Geometry: final body of the model. Coordinates: model frame, mm. A direction names the side the tool comes from. Coordinates: 2 decimals unless noted, no trailing zeros. Write each loop counter-clockwise with the first axis right and the second up, starting at its lowest first coordinate (ties: lowest second). Pieces come first, ordered by that corner, then holes. Notation, with made-up numbers: M 64,31 L 86,31 A10 ccw 86,35 Z; hole C 80.5,-11 d5. An arc over 180 degrees is marked long. Write item = value, one per line. Start each with the question number.
Item 1: Section C-C on x = 58. Output: boundary loops of the cut face in (y, z), plus the area to 3 significant figures.
Item 2: First-contact query: pin 1 Ø0.7 at (x, z) = (71, 1) entering from -Y; pin 2 Ø0.7 at (x, z) = (59.5, 1) entering from +Y; pin 3 Ø1.7 at (y, z) = (-13, -1) entering from +X. Flat tips, straight axial feed; report the tip coordinate or a pass-through.
Item 3: Section B-B on x = 8. Output: boundary loops of the cut face in (y, z), plus the area to 3 significant figures.
Item 4: Pull-direction query (X, two-part tool) for faces 1 (the flat face through (65, -30, 2)), 2 (the cylindrical face through (-15, -15, 2)), 3 (the cylindrical face through (35.369, -3.837, 2.465)); classes: +X half, -X half, draft (parallel to the pull), parting line (faces both ways), or undercut.
Item 5: Reachability of faces 4 (the flat face through (52, -15, -1)), 5 (the flat face through (68.43, -11.06, 3.62)), 6 (the cylindrical face through (16.5, -15.1, 4)), 7 (the flat face through (82, -21, -1)), 8 (the flat face through (60, -9, 1)) from +Z, -Z, +X, -X, +Y, -Y: full face, straight path, thin tool, end or side. Return the list, or none.
Item 6: Section D-D on x = 35. Output: boundary loops of the cut face in (y, z).
Item 7: Ray query, L1, parallel to Y at x = 63.1, z = 3.9; L2, parallel to Z at x = 16, y = -22.75; L3, parallel to Z at x = 73, y = -13.25. Return the intervals inside material, ascending. Write a range as [from, to].
Item 8: Section A-A on z = -1.25. Output: boundary loops of the cut face in (x, y), plus the area to 3 significant figures.
from build123d import *
from build123d.topology import SkipClean

# Parameters (mm, degrees)
BOSS_EXTRUDE1_DEPTH        = 5
CROQUIS3_W                 = 23
CROQUIS3_H                 = 12
CORTAR_EXTRUIR2_DEPTH      = 2.2
CORTAR_EXTRUIR3_DEPTH      = 91.182259896
CORTAR_EXTRUIR3_DEPTH_BACK = 91.182259896
CUT_EXTRUDE4_DEPTH         = 91.277350426
CUT_EXTRUDE4_DEPTH_BACK    = 2
CUT_EXTRUDE6_DEPTH         = 91.188691087
BOSS_EXTRUDE2_START        = 2.15
SKETCH9_W                  = 5
SKETCH9_H                  = 12
BOSS_EXTRUDE2_DEPTH        = 2.15
SKETCH10_R                 = 0.9
CUT_EXTRUDE7_DEPTH         = 8
CUT_EXTRUDE8_DEPTH         = 91.28578238


with BuildPart() as part:
    # Sketch1 → Boss-Extrude1 (new body)
    with BuildSketch(Plane(origin=(0, 0, 0), x_dir=(-1, 0, 0), z_dir=(0, 0, -1))):
        with BuildLine():
            Line((-70, 0), (-61, 0))
            ThreePointArc((-61, 0), (-35, -3.837363086), (-9, 0))
            Line((-9, 0), (0, 0))
            ThreePointArc((0, 0), (15, -15), (0, -30))
            Line((0, -30), (-9, -30))
            ThreePointArc((-9, -30), (-35, -26.162636914), (-61, -30))
            Line((-61, -30), (-70, -30))
            ThreePointArc((-70, -30), (-85, -15), (-70, 0))
        make_face()
        with BuildLine():
            Line((0, -11.4), (-5.4, -11.905))
            Line((-5.4, -11.905), (-5.4, -18.095))
            Line((-5.4, -18.095), (0, -18.6))
            ThreePointArc((0, -18.6), (3.6, -15), (0, -11.4))
        make_face(mode=Mode.SUBTRACT)
    extrude(amount=-BOSS_EXTRUDE1_DEPTH)

    # Croquis3 → Cortar-Extruir2 (cut)
    with BuildSketch(Plane(origin=(0, 0, 0), x_dir=(-1, 0, 0), z_dir=(0, 0, -1))):
        with Locations((-68.5, -15)):
            Rectangle(CROQUIS3_W, CROQUIS3_H)
    extrude(amount=-CORTAR_EXTRUIR2_DEPTH, mode=Mode.SUBTRACT)

    # Croquis4 → Cortar-Extruir3 (cut, two sides: drawn at the far end of the back side and taken through both)
    with BuildSketch(Plane(origin=(0, 0, 2.2), x_dir=(-1, 0, 0), z_dir=(0, 0, -1)).offset(-CORTAR_EXTRUIR3_DEPTH_BACK)):
        with BuildLine():
            Line((-66.2, -9.746429785), (-70.724590164, -12.416276944))
            ThreePointArc((-70.724590164, -12.416276944), (-72.2, -15), (-70.724590164, -17.583723056))
            Line((-70.724590164, -17.583723056), (-66.2, -20.253570215))
            ThreePointArc((-66.2, -20.253570215), (-57, -15), (-66.2, -9.746429785))
        make_face()
    extrude(amount=CORTAR_EXTRUIR3_DEPTH + CORTAR_EXTRUIR3_DEPTH_BACK, mode=Mode.SUBTRACT)

    # Sketch6 → Cut-Extrude4 (cut, two sides: drawn at the far end of the back side and taken through both)
    with BuildSketch(Plane.XY.offset(5).offset(-CUT_EXTRUDE4_DEPTH_BACK)):
        with BuildLine():
            Line((14.08705036, -12.406737159), (-1.12381295, -11.309587495))
            ThreePointArc((-1.12381295, -11.309587495), (-5.09, -15), (-1.12381295, -18.690412505))
            Line((-1.12381295, -18.690412505), (14.08705036, -17.593262841))
            ThreePointArc((14.08705036, -17.593262841), (16.5, -15), (14.08705036, -12.406737159))
        make_face()
    extrude(amount=CUT_EXTRUDE4_DEPTH + CUT_EXTRUDE4_DEPTH_BACK, mode=Mode.SUBTRACT)

    # Sketch8 → Cut-Extrude6 (cut, through all)
    with SkipClean():  # the faces are left unmerged after this step: merging them gives an invalid solid
        with BuildSketch(Plane.XY.offset(3)):
            with BuildLine():
                Line((-1.12381295, -11.309587495), (0, -11.4))
                ThreePointArc((0, -11.4), (-3.6, -15), (0, -18.6))
                Line((0, -18.6), (-1.12381295, -18.690412505))
                ThreePointArc((-1.12381295, -18.690412505), (-5.09, -15), (-1.12381295, -11.309587495))
            make_face()
        extrude(amount=-CUT_EXTRUDE6_DEPTH, mode=Mode.SUBTRACT)

    # Sketch9 → Boss-Extrude2 (add)
    with SkipClean():  # the faces are left unmerged after this step: merging them gives an invalid solid
        with BuildSketch(Plane(origin=(0, 0, 0), x_dir=(-1, 0, 0), z_dir=(0, 0, -1)).offset(BOSS_EXTRUDE2_START)):
            with BuildLine():
                Line((-83.747727085, -21), (-80, -21))
                Line((-80, -21), (-80, -9))
                Line((-80, -9), (-83.747727085, -9))
                ThreePointArc((-83.747727085, -9), (-85, -15), (-83.747727085, -21))
            make_face()
            with Locations((-54.5, -15)):
                Rectangle(SKETCH9_W, SKETCH9_H)
        extrude(amount=-BOSS_EXTRUDE2_DEPTH)

    # Sketch10 → Cut-Extrude7 (cut)
    with SkipClean():  # the faces are left unmerged after this step: merging them gives an invalid solid
        with BuildSketch(Plane(origin=(0, 0, -2.15), x_dir=(-1, 0, 0), z_dir=(0, 0, -1))):
            with Locations((-54.44, -15)):
                Circle(SKETCH10_R)
            with Locations((-82.56, -15)):
                Circle(SKETCH10_R)
        extrude(amount=-CUT_EXTRUDE7_DEPTH, mode=Mode.SUBTRACT)

    # Sketch11 → Cut-Extrude8 (cut, through all)
    with SkipClean():  # the faces are left unmerged after this step: merging them gives an invalid solid
        with BuildSketch(Plane.XY.offset(3)):
            with BuildLine():
                Line((5.4, -14.2), (14.9, -14.2))
                ThreePointArc((14.9, -14.2), (15.7, -15), (14.9, -15.8))
                Line((14.9, -15.8), (5.4, -15.8))
                Line((5.4, -15.8), (5.4, -14.2))
            make_face()
        extrude(amount=-CUT_EXTRUDE8_DEPTH, mode=Mode.SUBTRACT)


solid = part.part
Responses:
q1.outline = M -29.15,0 L -21,0 L -21,2.2 L -18.35,2.2 L -18.35,5 L -29.15,5 Z; M -11.65,2.2 L -9,2.2 L -9,0 L -0.85,0 L -0.85,5 L -11.65,5 Z
q1.area = 96.4 mm²
q2.pin_1 = -29.99
q2.pin_2 = -0.34
q2.pin_3 = 84.96
q3.outline = M -30,0 L -15.8,0 L -15.8,3 L -18.03,3 L -18.03,5 L -30,5 Z; M -14.2,0 L 0,0 L 0,5 L -11.97,5 L -11.97,3 L -14.2,3 Z
q3.area = 133 mm²
q4.face_1 = draft
q4.face_2 = -X half
q4.face_3 = undercut
q5.face_4 = -Z, -X, +Y, -Y
q5.face_5 = +Z, -Z
q5.face_6 = +Z
q5.face_7 = -Z, +X, -X, -Y
q5.face_8 = -Z
q6.outline = M -26.16,0 L -3.84,0 L -3.84,5 L -26.16,5 Z
q7.L1 = [-30, -21.1], [-8.9, 0]
q7.L2 = [0, 5]
q7.L3 = [2.2, 5]
q8.outline = M 52,-21 L 57,-21 L 57,-9 L 52,-9 Z; M 80,-21 L 83.75,-21 A15 ccw 83.75,-9 L 80,-9 Z; hole C 54.44,-15 d1.8; hole C 82.56,-15 d1.8
q8.area = 110 mm²
